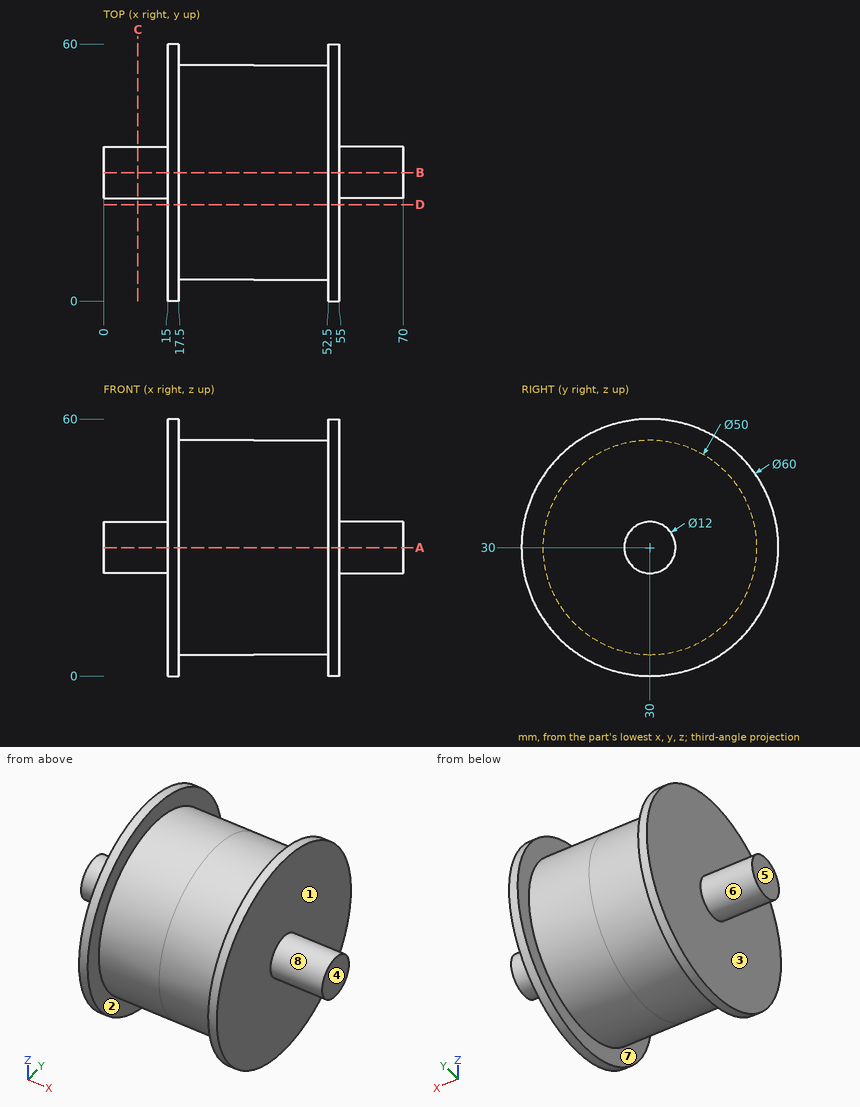
Here's the drawing with two shaded views (mm, measured from the low corner). I have some questions. A direction names the side the tool comes from. Give positions to 0.01 mm unless a question says otherwise; leave off trailing zeros. Order: outer loops, then holes, each group sorted by start corner. A loop starts at its lowest first (then second) coordinate and runs counter-clockwise, first axis right, second up. Notation, with made-up numbers: M -30,57.25 L -15,57.25 A32 cw -15,92.25 Z; hole C 75,41 d5. An arc over 180 degrees is marked long. One line per item, written item: value.
1) Please list where these lines run through material, in increasing order: line 1 along X through (y, z) = (4.5, 23); line 2 along X through (y, z) = (35.5, 27); line 3 along Z through (x, y) = (37, 11.5).
Answer sheet:
line 1: x = 15 to 17.5, 52.5 to 55
line 2: x = 15 to 55
line 3: z = 13.18 to 46.82
2) I want a section at A-A, the plane z = 30. List the corners of the cut face in (x, y) for me.
Answer sheet:
outline: M 0,24 L 15,24 L 15,0 L 17.5,0 L 17.5,5 L 52.5,5 L 52.5,0 L 55,0 L 55,24 L 70,24 L 70,36 L 55,36 L 55,60 L 52.5,60 L 52.5,55 L 17.5,55 L 17.5,60 L 15,60 L 15,36 L 0,36 Z
3) On a 3-axis mill with a long thin cutter (end or side, diameter ignored), from which of +Z, -Z, +X, -X, +Y, -Y can I reach the whole of each face in a straight line? I mean the marked faces 4, 5, 6, 7 and 8. Say none if no direction works.
Answer sheet:
face 4: +Z, -Z, +X, +Y, -Y
face 5: +Z, -Z, -X, +Y, -Y
face 6: -X
face 7: none
face 8: +X
4) I want a section at C-C, the plane x = 8. List the corners of the cut face in (y, z) for me, plus the area to 3 significant figures.
Answer sheet:
outline: C 30,30 d12
area: 113 mm^2
5) For P1, Ø8, axis at y = 14.5, z = 31.5, coming from the -X side; P2, Ø5, axis at y = 21.5, z = 42, coming from the +X side; P3, Ø1.5, axis at x = 61.5, z = 24, coming from the -Y side, each with a flat end and sliding along its axis, tell me the tip position at first contact or that it passes through.
Answer sheet:
P1: stops at x = 15
P2: stops at x = 55
P3: stops at y = 27.1
6) We'd pull the mould along X, two halves only. Please class the marked faces 1, 2 and 3: released by +X, released by -X, zero draft, split by the parting line, or undercut.
Answer sheet:
face 1: released by +X
face 2: undercut
face 3: released by -X
7) I want a section at D-D, the plane y = 22.5. List the corners of the cut face in (x, z) for me.
Answer sheet:
outline: M 15,0.95 L 17.5,0.95 L 17.5,6.15 L 52.5,6.15 L 52.5,0.95 L 55,0.95 L 55,59.05 L 52.5,59.05 L 52.5,53.85 L 17.5,53.85 L 17.5,59.05 L 15,59.05 Z
